The listing builds one solid part. Answer for the finished solid, in the listing's coordinates (mm). A direction names the side the tool comes from. Give positions to 0.01 mm unless a question says otherwise; leave off trailing zeros. Loops run counter-clockwise (first coordinate to the right, second up) from the corner with the lowest first, then second, coordinate; pieces in that order, holes last. Notation, with made-up numbers: M 41.25,59.25 L 67.25,59.25 A32 cw 67.25,91.25 Z; hole C -8.5,-4.75 d7. An arc over 180 degrees is marked long. Return JSON: item names as keys, results as strings.
from build123d import *

# Parameters (mm, degrees)
BOSS_EXTRUDE1_DEPTH = 20
SKETCH2_W           = 150
SKETCH2_H           = 20
SKETCH2_W_2         = 10
ROPEGROOVE1_DEPTH   = 0.5
SKETCH4_W           = 60
SKETCH4_H           = 20
ROPEGROOVE2_DEPTH   = 0.5
SKETCH5_W           = 30
SKETCH5_H           = 20
ROPEGROOVE3_DEPTH   = 0.5
SKETCH6_W           = 15
SKETCH6_H           = 5
CUT_EXTRUDE1_DEPTH  = 376.724633209
CUT_EXTRUDE2_DEPTH  = 377.065153929


with BuildPart() as part:
    # Sketch1 → Boss-Extrude1 (new body)
    with BuildSketch(Plane.XY):
        with BuildLine():
            Line((-8, 0), (-92, 0))
            ThreePointArc((-92, 0), (-100, 8), (-108, 0))
            Line((-108, 0), (-145, 0))
            Line((-145, 0), (-145, 13))
            Line((-145, 13), (-100, 20))
            Line((-100, 20), (0, 20))
            Line((0, 20), (350, 8))
            Line((350, 8), (375, 8))
            Line((375, 8), (375, 0))
            Line((375, 0), (8, 0))
            ThreePointArc((8, 0), (0, 8), (-8, 0))
        make_face()
    extrude(amount=BOSS_EXTRUDE1_DEPTH)

    # Sketch2 → RopeGroove1 (cut)
    with BuildSketch(Plane(origin=(0.684909168, 19.9765174, 0), x_dir=(0.9994127625749618, -0.03426558043114153, 0), z_dir=(0.034265580431141536, 0.9994127625749619, 0))):
        with Locations((149.314688391, -10)):
            Rectangle(SKETCH2_W, SKETCH2_H)
        with Locations((304.314688391, -10)):
            Rectangle(SKETCH2_W_2, SKETCH2_H)
    extrude(amount=-ROPEGROOVE1_DEPTH, mode=Mode.SUBTRACT)

    # Sketch4 → RopeGroove2 (cut)
    with BuildSketch(Plane(origin=(0, 20, 0), x_dir=(1, 0, 0), z_dir=(0, 1, 0))):
        with Locations((-50, -10)):
            Rectangle(SKETCH4_W, SKETCH4_H)
    extrude(amount=-ROPEGROOVE2_DEPTH, mode=Mode.SUBTRACT)

    # Sketch5 → RopeGroove3 (cut)
    with BuildSketch(Plane(origin=(-5.400192864, 34.715525554, 0), x_dir=(0.9881164689548824, 0.15370700628187053, 0), z_dir=(-0.15370700628187053, 0.9881164689548824, 0))):
        with Locations((-123.278696917, -10)):
            Rectangle(SKETCH5_W, SKETCH5_H)
    extrude(amount=-ROPEGROOVE3_DEPTH, mode=Mode.SUBTRACT)

    # Sketch6 → Cut-Extrude1 (cut, through all)
    with BuildSketch(Plane(origin=(0, 8, 0), x_dir=(1, 0, 0), z_dir=(0, 1, 0))):
        with Locations((367.5, -10)):
            Rectangle(SKETCH6_W, SKETCH6_H)
    extrude(amount=-CUT_EXTRUDE1_DEPTH, mode=Mode.SUBTRACT)

    # Sketch7 → Cut-Extrude2 (cut, through all)
    with BuildSketch(Plane.XY.offset(20)):
        with BuildLine():
            ThreePointArc((364, 4), (365, 3), (366, 4))
            Line((366, 4), (364, 4))
        make_face()
        with BuildLine():
            Line((364, 4), (366, 4))
            ThreePointArc((366, 4), (365, 5), (364, 4))
        make_face()
        with BuildLine():
            ThreePointArc((370, 4), (371, 3), (372, 4))
            Line((372, 4), (370, 4))
        make_face()
        with BuildLine():
            Line((370, 4), (372, 4))
            ThreePointArc((372, 4), (371, 5), (370, 4))
        make_face()
    extrude(amount=-CUT_EXTRUDE2_DEPTH, mode=Mode.SUBTRACT)


solid = part.part
(1) Given pin 1 (3 mm diameter, centred on x = 371, y = 4, fed in from +Z); pin 2 (2.5 mm diameter, centred on y = 4.5, z = 11, fed in from +X); pin 3 (5 mm diameter, centred on x = 115, z = 17.5, fed in from +Y); pin 4 (3 mm diameter, centred on x = 140.5, z = 3.5, fed in from +Y), each flat-ended and moving along its own axis, determine where each tip first touches the part or whether it passes through.
Values follow:
{"pin 1": "z = 20", "pin 2": "x = 360", "pin 3": "y = 15.64", "pin 4": "y = 14.73"}
(2) Straight lines are drawn through the part: line 1 along Y through (x, z) = (371, 5.5); line 2 along X through (y, z) = (2.5, 17); line 3 along Y through (x, z) = (255, 18.5). For each, find the intervals that lie inside material, in ascending order.
Values follow:
{"line 1": "0 to 3, 5 to 8", "line 2": "-145 to -107.6, -92.4 to -7.6, 7.6 to 375", "line 3": "0 to 11.26"}
(3) The part is cut by section B-B (x = 214.5). Determine the outline of the cut face in (y, z).
Values follow:
{"outline": "M 0,0 L 12.15,0 L 12.15,20 L 0,20 Z"}
(4) The part is cut by section A-A (x = 82). Determine the outline of the cut face in (y, z).
Values follow:
{"outline": "M 0,0 L 16.69,0 L 16.69,20 L 0,20 Z"}
(5) Determine the mould class of faces 1 (the flat face through (359.5, 8, 9.9)), 2 (the cylindrical face through (0, 8, 10)), 3 (the flat face through (-106.283, 19.023, 9.86)) for opening direction X: released by +X, released by -X, zero draft, split by the parting line, or undercut.
Values follow:
{"face 1": "zero draft", "face 2": "undercut", "face 3": "released by -X"}
(6) A tool of negligible diameter and unlimited length cuts with its end or side. For faces 4 (the flat face through (367, 4, 7.5)), 5 (the flat face through (-50, 19.5, 10)), 6 (the flat face through (-145, 6, 10)), from which of +Z, -Z, +X, -X, +Y, -Y can it reach the whole face along a straight path? Write none if from no direction.
Values follow:
{"face 4": "+X, +Y, -Y", "face 5": "+Z, -Z, +Y", "face 6": "+Z, -Z, -X, +Y, -Y"}
